Input: part model. Units: mm. Frame: model coordinates. A direction names the side the tool comes from. Round coordinates to 2 decimals unless told otherwise and drop trailing zeros. Loops run counter-clockwise (first coordinate to the right, second up) from the corner with the lowest first, then second, coordinate; pieces in that order, holes last. Notation, with made-up numbers: (-5, -36.75) - (26, -36.75) arc R30 cw to (26, -7.75) - close; hole circle Ø3 at (65, 58). An arc over 180 degrees is marked (long way). Use CSV: the item, a comma, the result in double quotes. Start each with the question number.
1. Access query for faces 1 (the flat face through (5, 0, 0)), 2 (the flat face through (-8.4, 9.4, 27.65)), 3 (the flat face through (0, 3.1, 33.5)), 4 (the flat face through (0, 2.6, 17)). Directions: +Z, -Z, +X, -X, +Y, -Y. A direction counts if a zero-diameter tool reaches every point of the face in a straight line with its end or side. Return the directions, or none.
2. Material intervals for probe 1 along Y at (x, z) = (0, 22); probe 2 along Y at (x, z) = (-1.5, 14); probe 3 along X at (y, z) = (-1.25, 26), sorted ascending. Write a range as from..to.
3. Cut plane A-A (y = 0). Return loops of the section in (x, z), and give its area (3 significant figures).
4. Cut plane C-C (z = 28.5). Return loops of the section in (x, y).
5. Cut plane D-D (z = 17.5). Return loops of the section in (x, y).
6. Pull-direction query (X, two-part tool) for faces 5 (the cylindrical face through (11.18, -4.63, 14.14)), 6 (the flat face through (2.9, 3.3, 34)), 7 (the conical face through (0.1, -3.3, 33.2)); classes: +X half, -X half, draft (parallel to the pull), parting line (faces both ways), or undercut.
7. Pin query (flat end, axial travel): P1, Ø1, axis at x = 0, z = 24, coming from the -Y side; P2, Ø12, axis at y = -1, z = 14, coming from the +X side; P3, Ø5.5, axis at x = 0, y = 0, coming from the -Z side. Return the tip coordinate at first contact, or that it passes through.
8. Cut plane B-B (x = 0). Return loops of the section in (y, z).
```python
from build123d import *

# Parameters (mm, degrees)
SKETCH2_R           = 12.1
BOSS_EXTRUDE1_DEPTH = 34
BOSS_EXTRUDE2_START = -6.35
SKETCH3_R           = 14
SKETCH3_R_2         = 12.1
BOSS_EXTRUDE2_DEPTH = 6.35
CHAMFER1_SIZE       = 1


with BuildPart() as part:
    # Sketch2 → Boss-Extrude1 (new body)
    with BuildSketch(Plane.XY):
        Circle(SKETCH2_R)
        with BuildLine():
            Line((-1.688194302, 2.6), (1.688194302, 2.6))
            ThreePointArc((1.688194302, 2.6), (0, -3.1), (-1.688194302, 2.6))
        make_face(mode=Mode.SUBTRACT)
    extrude(amount=BOSS_EXTRUDE1_DEPTH)

    # Sketch3 → Boss-Extrude2 (add)
    # profile 1 of 2: a face of its own
    with BuildSketch(Plane.XY.offset(34).offset(BOSS_EXTRUDE2_START)):
        Circle(SKETCH3_R)
        Circle(SKETCH3_R_2, mode=Mode.SUBTRACT)
    # profile 2 of 2: a face of its own
    with BuildSketch(Plane.XY.offset(34).offset(BOSS_EXTRUDE2_START)):
        Circle(SKETCH3_R_2)
        with BuildLine():
            Line((-1.688194302, 2.6), (1.688194302, 2.6))
            ThreePointArc((1.688194302, 2.6), (0, -3.1), (-1.688194302, 2.6))
        make_face(mode=Mode.SUBTRACT)
    extrude(amount=BOSS_EXTRUDE2_DEPTH)

    # Chamfer1
    chamfer1_edges = [part.edges().sort_by_distance(p)[0] for p in [
        (0, 2.6, 34),
        (-12.1, 0, 0),
        (0, 2.6, 0),
        (0, -3.1, 0),
        (0, -3.1, 34),
    ]]
    chamfer(chamfer1_edges, length=CHAMFER1_SIZE)


solid = part.part
```
Established:
1,face 1,"-Z, +X, -X, +Y, -Y"
1,face 2,"-Z"
1,face 3,"+Z"
1,face 4,"+Z, -Z"
2,probe 1,"y = -12.1..-3.1, 2.6..12.1"
2,probe 2,"y = -12.01..-2.71, 2.6..12.01"
2,probe 3,"x = -12.04..-2.84, 2.84..12.04"
3,outline,"(-14, 27.65) - (-12.1, 27.65) - (-12.1, 1) - (-11.1, 0) - (-4.1, 0) - (-3.1, 1) - (-3.1, 33) - (-4.1, 34) - (-14, 34) - close; (3.1, 1) - (4.1, 0) - (11.1, 0) - (12.1, 1) - (12.1, 27.65) - (14, 27.65) - (14, 34) - (4.1, 34) - (3.1, 33) - close"
3,area,"633 mm2"
4,outline,"circle Ø28 at (0, 0); hole (-1.69, 2.6) arc R3.1 ccw (long way) to (1.69, 2.6) - close"
5,outline,"circle Ø24.2 at (0, 0); hole (-1.69, 2.6) arc R3.1 ccw (long way) to (1.69, 2.6) - close"
6,face 5,"parting line"
6,face 6,"draft"
6,face 7,"undercut"
7,P1,"stops at y = -12.1"
7,P2,"stops at x = 12.1"
7,P3,"stops at z = 0.85"
8,outline,"(-14, 27.65) - (-12.1, 27.65) - (-12.1, 1) - (-11.1, 0) - (-4.1, 0) - (-3.1, 1) - (-3.1, 33) - (-4.1, 34) - (-14, 34) - close; (2.6, 1) - (3.6, 0) - (11.1, 0) - (12.1, 1) - (12.1, 27.65) - (14, 27.65) - (14, 34) - (3.6, 34) - (2.6, 33) - close"
